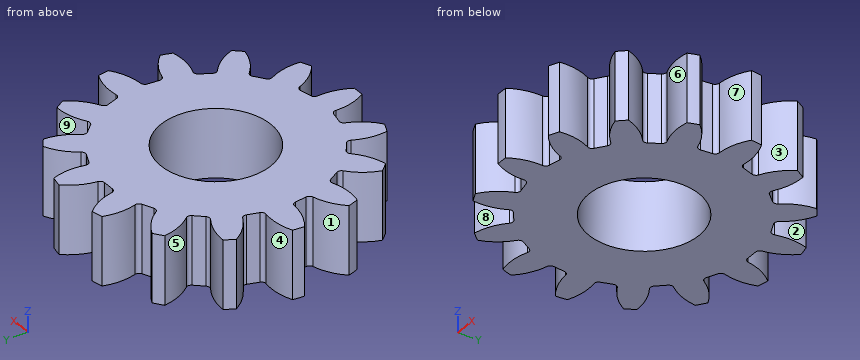
from build123d import *

# Parameters (mm, degrees)
SKETCH1_R                = 6.335999901
BOSS_EXTRUDE1_DEPTH      = 1.524
CUT_EXTRUDE1_DEPTH       = 10.089134474
FILLET1_R                = 0.191999997
CIRPATTERN1_COUNT        = 15
FILLET1_OF_CIRPATTERN1_R = 0.191999997
CUT_EXTRUDE2_DEPTH       = 10.455482489
CUT_EXTRUDE2_DEPTH_BACK  = 10.455482489
SKETCH4_R                = 2.45


with BuildPart() as part:
    # Sketch1 → Boss-Extrude1 (new, symmetric)
    with BuildSketch(Plane.XY):
        with Locations(Location((0, 0, 0), (0, 0, 180))):
            Circle(SKETCH1_R)
    extrude(amount=BOSS_EXTRUDE1_DEPTH, both=True)

    # Sketch3 → Cut-Extrude1 (cut, symmetric)
    with BuildSketch(Plane.XY):
        with BuildLine():
            Line((-0.428414679, 4.780843037), (0.428414679, 4.780843037))
            ThreePointArc((0.428414679, 4.780843037), (1.010780942, 6.170659573), (2.288190337, 6.970012879))
            ThreePointArc((2.288190337, 6.970012879), (0, 7.335999901), (-2.288190337, 6.970012879))
            ThreePointArc((-2.288190337, 6.970012879), (-1.010780942, 6.170659573), (-0.428414679, 4.780843037))
        make_face()
    cut_extrude1 = extrude(amount=CUT_EXTRUDE1_DEPTH, both=True, mode=Mode.SUBTRACT)

    # Fillet1
    fillet1_edges = [part.edges().sort_by_distance(p)[0] for p in [
        (-0.428414679, 4.780843037, 0),
        (0.428414679, 4.780843037, 0),
    ]]
    fillet(fillet1_edges, radius=FILLET1_R)

    # CirPattern1: Cut-Extrude1 ×15 about axis
    cirpattern1_axis = Axis((0, 0, 0), (0, 0, 1))
    for i in range(1, CIRPATTERN1_COUNT):
        add(cut_extrude1.rotate(cirpattern1_axis, i * 360 / CIRPATTERN1_COUNT), mode=Mode.SUBTRACT)

    # Fillet1 of CirPattern1
    fillet1_of_cirpattern1_edges = [part.edges().sort_by_distance(p)[0] for p in [
        (-2.335920332, 4.193265492, 0),
        (-1.553167764, 4.541769388, 0),
        (-3.839524138, 2.880634248, 0),
        (-3.26619339, 3.517382552, 0),
        (-4.67923934, 1.069915174, 0),
        (-4.414464507, 1.884808318, 0),
        (-4.70987155, -0.925801954, 0),
        (-4.799434606, -0.073666397, 0),
        (-3.926124182, -2.761439514, 0),
        (-4.354538861, -2.019403523, 0),
        (-2.463514275, -4.119599094, 0),
        (-3.156703787, -3.615967434, 0),
        (-0.574940369, -4.765442566, 0),
        (-1.41304595, -4.587297726, 0),
        (1.41304595, -4.587297726, 0),
        (0.574940369, -4.765442566, 0),
        (3.156703787, -3.615967434, 0),
        (2.463514275, -4.119599094, 0),
        (4.354538861, -2.019403523, 0),
        (3.926124182, -2.761439514, 0),
        (4.799434606, -0.073666397, 0),
        (4.70987155, -0.925801954, 0),
        (4.414464507, 1.884808318, 0),
        (4.67923934, 1.069915174, 0),
        (3.26619339, 3.517382552, 0),
        (3.839524138, 2.880634248, 0),
        (1.553167764, 4.541769388, 0),
        (2.335920332, 4.193265492, 0),
    ]]
    fillet(fillet1_of_cirpattern1_edges, radius=FILLET1_OF_CIRPATTERN1_R)

    # Sketch4 → Cut-Extrude2 (cut, two sides: drawn at the far end of the back side and taken through both)
    with BuildSketch(Plane.XY.offset(1.524).offset(-CUT_EXTRUDE2_DEPTH_BACK)):
        Circle(SKETCH4_R)
    extrude(amount=CUT_EXTRUDE2_DEPTH + CUT_EXTRUDE2_DEPTH_BACK, mode=Mode.SUBTRACT)


solid = part.part
Build history of the part. All positions in model axes, mm. Face numbers are marked on the shaded views. A direction names the side the tool comes from. Round coordinates to 2 decimals unless told otherwise and drop trailing zeros. Write each loop counter-clockwise with the first axis right and the second up, starting at its lowest first coordinate (ties: lowest second). Pieces come first, ordered by that corner, then holes. Notation, with made-up numbers: M 33,75.25 L 44,75.25 A31 ccw 44,104.25 Z; hole C 8.25,20 d11. An arc over 180 degrees is marked long. Answer as a JSON object with one key per item and string values. Group by question number.
(1) Flat gauge pins, fed straight in: pin 1 (1 mm diameter, centred on y = -2.5, z = 0, fed in from +X); pin 2 (1 mm diameter, centred on y = 1, z = 0, fed in from -X); pin 3 (4.5 mm diameter, centred on x = 0, y = 0, fed in from +Z). Where does each tip first touch, or does it go through?
(2) Cut at B-B (y = -5.25). Give the cut face in (x, z).
(3) Which spindle directions (+Z, -Z, +X, -X, +Y, -Y) get a long thin tool onto all of the face, cutting with end or side? Do the marked faces 5, 6, 7, 8 and 9. Say none if no direction does.
(4) Cut at A-A (x = 0). Give the cut face in (y, z).
(5) Drill centre lines: L1, parallel to Y at x = 0, z = -0.35; L2, parallel to X at y = 3, z = -0.45; L3, parallel to Y at x = -5, z = 0.3. Where is each one in solid material? Low to high.
(6) Cut at D-D (y = 2.75). Give the cut face in (x, z), and give its area (3 significant figures).
(7) Cut at C-C (y = 0.75). Give the cut face in (x, z), and give its area (3 significant figures).
(8) Mould opens along X. For the marked faces 1, 2, 3 and 4 say: pulls with the +X half, pulls with the -X half, needs draft (parallel to the pull), parting line crosses it, or undercut.
Responses:
{
 "1": {"pin 1": "stops at x = 6.01", "pin 2": "stops at x = -6.32", "pin 3": "passes through"},
 "2": {"outline": "M -2.81,-1.52 L -1.73,-1.52 L -1.73,1.52 L -2.81,1.52 Z; M -0.59,-1.52 L 0.59,-1.52 L 0.59,1.52 L -0.59,1.52 Z; M 1.73,-1.52 L 2.81,-1.52 L 2.81,1.52 L 1.73,1.52 Z"},
 "3": {"face 5": "+Z, -Z, -X", "face 6": "+Z, -Z", "face 7": "+Z, -Z, +X", "face 8": "+Z, -Z, -Y", "face 9": "+Z, -Z, +Y"},
 "4": {"outline": "M -6.34,-1.52 L -2.45,-1.52 L -2.45,1.52 L -6.34,1.52 Z; M 2.45,-1.52 L 4.78,-1.52 L 4.78,1.52 L 2.45,1.52 Z"},
 "5": {"L1": "y = -6.34 to -2.45, 2.45 to 4.78", "L2": "x = -5.58 to -4.01, -3.73 to 3.73, 4.01 to 5.58", "L3": "y = -2.22 to -1, -0.07 to 1.12, 2.24 to 3.36"},
 "6": {"outline": "M -5.48,-1.52 L 5.48,-1.52 L 5.48,1.52 L -5.48,1.52 Z", "area": "33.4 mm2"},
 "7": {"outline": "M -6.29,-1.52 L -2.33,-1.52 L -2.33,1.52 L -6.29,1.52 Z; M 2.33,-1.52 L 6.29,-1.52 L 6.29,1.52 L 2.33,1.52 Z", "area": "24.1 mm2"},
 "8": {"face 1": "pulls with the -X half", "face 2": "undercut", "face 3": "pulls with the +X half", "face 4": "undercut"}
}
